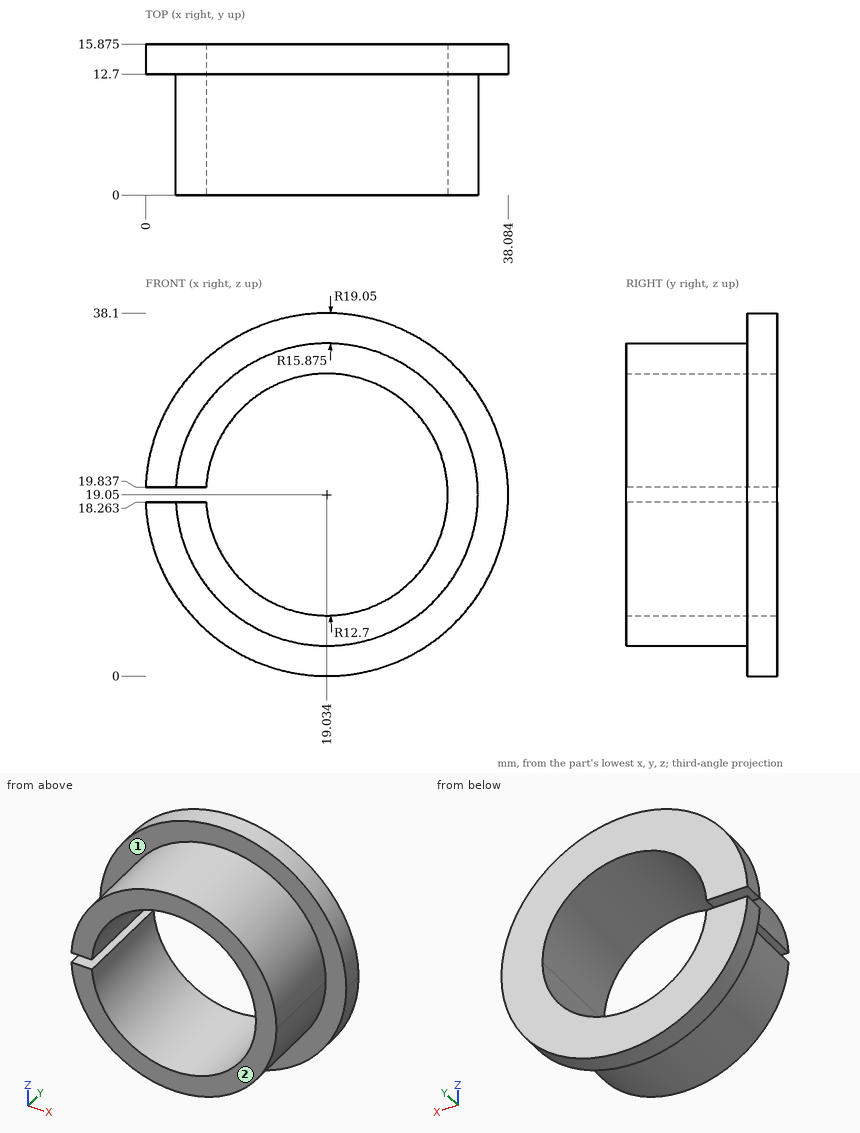
The figure shows three views and two pictorial views of one solid part (mm, origin at its lowest corner). Answer the questions. A direction names the side the tool comes from. Coordinates: 2 decimals unless noted, no trailing zeros. Answer as a JSON object with one key per item and string values.
Q1. A tool of negligible diameter and unlimited length cuts with its end or side. For the marked faces 1 and 2, from which of +Z, -Z, +X, -X, +Y, -Y can it reach the whole face along a straight path? Write none if from no direction.
The answers:
{"face 1": "-Y", "face 2": "+Z, -Z, +X, -X, -Y"}
Q2. Consider line 1 (Y direction, x = 11, z = 35.5) (1 decimal); line 2 (X direction, y = 5, z = 28) (1 decimal); line 3 (X direction, y = 12.5, z = 8.5) (1 decimal). Determine where each line is inside the solid, lowest interval first. Write a range as [from, to].
The answers:
{"line 1": "y = [12.7, 15.9]", "line 2": "x = [5.9, 10], [28, 32.1]", "line 3": "x = [7.2, 12], [26.1, 30.9]"}
Q3. Flat-ended cylindrical pins translate along their axes: pin 1 Ø8 at (x, z) = (11, 28) entering from -Y; pin 2 Ø2 at (y, z) = (14, 21.5) entering from +X; pin 3 Ø2 at (x, y) = (5, 10) entering from -Z (1 decimal); pin 4 Ø7 at (x, y) = (2, 4.5) entering from +Z. Find the tip coordinate at first contact, or state that the pin passes through.
The answers:
{"pin 1": "stops at y = 0", "pin 2": "stops at x = 38.03", "pin 3": "stops at z = 10", "pin 4": "stops at z = 27.35"}
